```python
from build123d import *

# Parameters (mm, degrees)
SKETCH1_R           = 1.5
BOSS_EXTRUDE2_DEPTH = 6


with BuildPart() as part:
    # Sketch1 → Boss-Extrude2 (new body)
    # profile 1 of 2: a face of its own
    with BuildSketch(Plane.XY):
        with BuildLine():
            Line((-7.766144764, 8.750016816), (-7.766144764, -18))
            Line((-7.766144764, -18), (7.733855236, -18))
            Line((7.733855236, -18), (7.733855236, 8.750016816))
            ThreePointArc((7.733855236, 8.750016816), (7.327886817, 11.225436), (6.152513266, 13.44151531))
            ThreePointArc((6.152513266, 13.44151531), (-2.491563947, 16.094048398), (-7.766144764, 8.750016816))
        make_face()
        with Locations((-0.016144764, -6.375)):
            Circle(SKETCH1_R, mode=Mode.SUBTRACT)
        with Locations((-0.016144764, 11.125)):
            Circle(SKETCH1_R, mode=Mode.SUBTRACT)
    # profile 2 of 2: a face of its own
    with BuildSketch(Plane.XY):
        with BuildLine():
            ThreePointArc((10.704360482, -18), (11.593820566, -18.542987134), (11.517349886, -19.582278481))
            ThreePointArc((11.517349886, -19.582278481), (0, -25.5), (-11.517349886, -19.582278481))
            ThreePointArc((-11.517349886, -19.582278481), (-11.593820566, -18.542987134), (-10.704360482, -18))
            Line((-10.704360482, -18), (10.704360482, -18))
        make_face()
    extrude(amount=BOSS_EXTRUDE2_DEPTH)


solid = part.part
```
Build history of the part. All positions in model axes, mm. A direction names the side the tool comes from. Round coordinates to 2 decimals unless told otherwise and drop trailing zeros. Write each loop counter-clockwise with the first axis right and the second up, starting at its lowest first coordinate (ties: lowest second). Pieces come first, ordered by that corner, then holes. Notation, with made-up numbers: (51.25, -21.5) - (96.25, -21.5) arc R15 cw to (96.25, 5.5) - close; hole circle Ø11 at (48.25, 30). An arc over 180 degrees is marked (long way). Write each question's results on one line, items separated by ' | '. Start each with the question number.
Item 1: Saw through at C-C (y = -14). Write the cut outline in (x, z), and give its area (3 significant figures).
Item 2: Mould opens along X. For faces 1 (the face through (7.734, -5, 3)), 2 (the face through (-9, -18, 3)), 3 (the face through (-0.34, -7.84, 2.96)) say: pulls with the +X half, pulls with the -X half, needs draft (parallel to the pull), parting line crosses it, or undercut.
Item 3: Saw through at B-B (z = 5.2). Write the cut outline in (x, y) (3 decimals), and give its area (3 significant figures).
Item 4: Which spindle directions (+Z, -Z, +X, -X, +Y, -Y) get a long thin tool onto all of the face, cutting with end or side? Do faces 4 (the face through (9, -18, 3)), 5 (the face through (-0.34, 9.66, 2.96)), 6 (the face through (-7.766, -4, 3)). Say none if no direction does.
Item 5: Saw through at A-A (x = -0.25). Write the cut outline in (y, z), and give its area (3 significant figures).
Item 6: Saw through at D-D (x = -6.5). Write the cut outline in (y, z).
Item 7: Drop flat-ended pins along their axis: P1, Ø1.8, axis at y = -7.5, z = 2.5, coming from the -X side; P2, Ø0.9, axis at x = -9.5, z = 2, coming from the +Y side; P3, Ø3, axis at x = -5, z = 4, coming from the -Y side. Give the stop position or say it passes through.
Item 8: Wall check: L1, parallel to Y at x = 0.25, z = 3.05; L2, parallel to X at y = -0.5, z = 5.7; L3, parallel to X at y = 10, z = 4.7. Give the ranges that are in metal, low to high. Write a range as [from, to].
Results are:
1) outline: (-7.77, 0) - (7.73, 0) - (7.73, 6) - (-7.77, 6) - close | area: 93.0 mm²
2) face 1: pulls with the +X half | face 2: needs draft | face 3: undercut
3) outline: (-11.517, -19.582) arc R14.167 ccw to (11.517, -19.582) arc R1 ccw to (10.704, -18) - (7.734, -18) - (7.734, 8.75) arc R7.75 ccw to (-7.766, 8.75) - (-7.766, -18) - (-10.704, -18) arc R1 ccw to start; hole circle Ø3 at (-0.016, -6.375); hole circle Ø3 at (-0.016, 11.125) | area: 627 mm²
4) face 4: +Z, -Z, +X, +Y | face 5: +Z, -Z | face 6: +Z, -Z, -X, +Y
5) outline: (-25.5, 0) - (-7.86, 0) - (-7.86, 6) - (-25.5, 6) - close; (-4.89, 0) - (9.64, 0) - (9.64, 6) - (-4.89, 6) - close; (12.61, 0) - (16.5, 0) - (16.5, 6) - (12.61, 6) - close | area: 216 mm²
6) outline: (-23.92, 0) - (13, 0) - (13, 6) - (-23.92, 6) - close
7) P1: stops at x = -7.77 | P2: stops at y = -18 | P3: stops at y = -25.06
8) L1: y = [-25.5, -7.85], [-4.9, 9.65], [12.6, 16.5] | L2: x = [-7.77, 7.73] | L3: x = [-7.66, -1.01], [0.98, 7.63]
